Input: part model. Units: mm. Frame: model coordinates. Face numbers are marked on the shaded views. A direction names the side the tool comes from. Give positions to 0.01 mm unless a question says otherwise; leave off trailing zeros. Loops run counter-clockwise (first coordinate to the right, second up) from the corner with the lowest first, then second, coordinate; pieces in that order, holes last. Notation, with made-up numbers: (74.25, 3) - (115.25, 3) arc R26 cw to (115.25, 18) - close; hole circle Ø9 at (14, -13.5). An arc over 180 degrees is marked (long way). Answer as a JSON object with one key per item and string values.
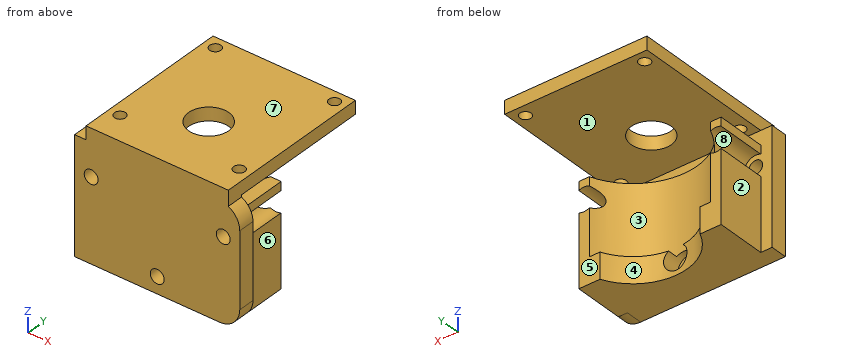
from build123d import *

# Parameters (mm, degrees)
SKETCH_1_W          = 30
SKETCH_1_H          = 30
EXTRUDE_1_DEPTH     = 5
SKETCH_2_W          = 30
SKETCH_2_H          = 5
EXTRUDE_2_DEPTH     = 10
SKETCH_3_R          = 2.1
CUT_EXTRUDE_1_DEPTH = 5
EXTRUDE_3_DEPTH     = 20
SKETCH_5_W          = 35
SKETCH_5_H          = 5
EXTRUDE_4_DEPTH     = 10
SKETCH_6_W          = 35
SKETCH_6_H          = 5
EXTRUDE_5_DEPTH     = 10
SKETCH_7_R          = 2.1
CUT_EXTRUDE_2_DEPTH = 10
FILLET_1_R          = 6.17
FILLET_2_R          = 6.17
SKETCH_8_W          = 43.093455854
SKETCH_8_H          = 31.755969384
CUT_EXTRUDE_3_DEPTH = 25
SKETCH_9_W          = 43.1
SKETCH_9_H          = 43.1
SKETCH_9_R          = 6.1
SKETCH_9_R_2        = 1.7
EXTRUDE_6_DEPTH     = 4
EXTRUDE_7_DEPTH     = 23
EXTRUDE_8_DEPTH     = 7.8
CUT_EXTRUDE_START   = -35
SKETCH_12_W         = 51.858978503
SKETCH_12_H         = 9.121001398
CUT_EXTRUDE_4_DEPTH = 35
SKETCH_14_W         = 43.1
SKETCH_14_H         = 5
EXTRUDE_9_DEPTH     = 8.2
SKETCH_15_R         = 2.1
CUT_EXTRUDE_5_DEPTH = 49.1
SKETCH_16_R         = 3.55
CUT_EXTRUDE_6_DEPTH = 44.1


with BuildPart() as part:
    # Sketch 1 → Extrude 1 (new body)
    with BuildSketch(Plane.XY):
        Rectangle(SKETCH_1_W, SKETCH_1_H)
    extrude(amount=EXTRUDE_1_DEPTH)

    # Sketch 2 → Extrude 2 (add)
    with BuildSketch(Plane(origin=(0, 0, 0), x_dir=(-1, 0, 0), z_dir=(0, 0, -1))):
        with Locations((0, -12.5)):
            Rectangle(SKETCH_2_W, SKETCH_2_H)
    extrude(amount=EXTRUDE_2_DEPTH)

    # Sketch 3 → Cut-Extrude 1 (cut)
    with BuildSketch(Plane(origin=(0, -10, 0), x_dir=(1, 0, 0), z_dir=(0, 1, 0))):
        with Locations((0, 5)):
            Circle(SKETCH_3_R)
    extrude(amount=-CUT_EXTRUDE_1_DEPTH, mode=Mode.SUBTRACT)

    # Sketch 4 → Extrude 3 (add)
    with BuildSketch(Plane.XY.offset(5)):
        Polygon((10.2, -15), (15, -15), (15, 15), (-15, 15), (-15, -15), (-10.2, -15), (-10.2, -18.997175384), (10.2, -18.997175384), align=None)
    extrude(amount=EXTRUDE_3_DEPTH)

    # Sketch 5 → Extrude 4 (add)
    with BuildSketch(Plane.ZY.offset(15)):
        with Locations((7.5, -12.5)):
            Rectangle(SKETCH_5_W, SKETCH_5_H)
    extrude(amount=EXTRUDE_4_DEPTH)

    # Sketch 6 → Extrude 5 (add)
    with BuildSketch(Plane(origin=(15, 0, 0), x_dir=(0, 0, -1), z_dir=(1, 0, 0))):
        with Locations((-7.5, -12.5)):
            Rectangle(SKETCH_6_W, SKETCH_6_H)
    extrude(amount=EXTRUDE_5_DEPTH)

    # Sketch 7 → Cut-Extrude 2 (cut)
    with BuildSketch(Plane(origin=(0, -10, 0), x_dir=(1, 0, 0), z_dir=(0, 1, 0))):
        with Locations((-20, -15)):
            Circle(SKETCH_7_R)
        with Locations((20, -15)):
            Circle(SKETCH_7_R)
    extrude(amount=-CUT_EXTRUDE_2_DEPTH, mode=Mode.SUBTRACT)

    # Fillet 1
    fillet_1_edges = [part.edges().sort_by_distance(p)[0] for p in [
        (25, -12.5, 25),
    ]]
    fillet(fillet_1_edges, radius=FILLET_1_R)

    # Fillet 2
    fillet_2_edges = [part.edges().sort_by_distance(p)[0] for p in [
        (25, -12.5, -10),
    ]]
    fillet(fillet_2_edges, radius=FILLET_2_R)

    # Sketch 8 → Cut-Extrude 3 (cut)
    with BuildSketch(Plane(origin=(0, 15, 0), x_dir=(1, 0, 0), z_dir=(0, 1, 0))):
        with Locations((-0.577881592, -10.851708682)):
            Rectangle(SKETCH_8_W, SKETCH_8_H)
    extrude(amount=-CUT_EXTRUDE_3_DEPTH, mode=Mode.SUBTRACT)

    # Sketch 12 → Cut-Extrude 4 (cut)
    with BuildSketch(Plane.XY.offset(25).offset(CUT_EXTRUDE_START)):
        with Locations((0.929489252, -19.560500699)):
            Rectangle(SKETCH_12_W, SKETCH_12_H)
    extrude(amount=CUT_EXTRUDE_4_DEPTH, mode=Mode.SUBTRACT)



with BuildPart() as body_2:
    # Sketch 9 → Extrude 6 (new body)
    with BuildSketch(Plane.XY.offset(29)):
        with Locations((0, 11.55)):
            Rectangle(SKETCH_9_W, SKETCH_9_H)
        with Locations((0, 4.5)):
            Circle(SKETCH_9_R, mode=Mode.SUBTRACT)
        with Locations((18.05, 29.6)):
            Circle(SKETCH_9_R_2, mode=Mode.SUBTRACT)
        with Locations((18.05, -6.5)):
            Circle(SKETCH_9_R_2, mode=Mode.SUBTRACT)
        with Locations((-18.05, -6.5)):
            Circle(SKETCH_9_R_2, mode=Mode.SUBTRACT)
        with Locations((-18.05, 29.6)):
            Circle(SKETCH_9_R_2, mode=Mode.SUBTRACT)
    extrude(amount=-EXTRUDE_6_DEPTH)


with BuildPart() as body_3:
    # Sketch 10 → Extrude 7 (new body)
    with BuildSketch(Plane(origin=(0, 0, 20.8), x_dir=(-1, 0, 0), z_dir=(0, 0, -1))):
        with BuildLine():
            Line((-21.55, 5), (-18.367022078, 5))
            ThreePointArc((-18.367022078, 5), (0, -7.95), (18.367022078, 5))
            Line((18.367022078, 5), (21.55, 5))
            Line((21.55, 5), (21.55, -10))
            Line((21.55, -10), (-21.55, -10))
            Line((-21.55, -10), (-21.55, 5))
        make_face()
    extrude(amount=EXTRUDE_7_DEPTH)

    # Sketch 11 → Extrude 8 (add)
    with BuildSketch(Plane(origin=(0, 0, -2.2), x_dir=(-1, 0, 0), z_dir=(0, 0, -1))):
        with BuildLine():
            Line((-21.55, 5), (-15.144223321, 5))
            ThreePointArc((-15.144223321, 5), (0, -4.95), (15.144223321, 5))
            Line((15.144223321, 5), (21.55, 5))
            Line((21.55, 5), (21.55, -10))
            Line((21.55, -10), (-21.55, -10))
            Line((-21.55, -10), (-21.55, 5))
        make_face()
    extrude(amount=EXTRUDE_8_DEPTH)


with BuildPart() as part_1:
    add(part.part)

    add(body_2.part)  # Extrude 9 merges body 2

    add(body_3.part)  # Extrude 9 merges body 3
    # Sketch 14 → Extrude 9 (add)
    with BuildSketch(Plane.XY.offset(29)):
        with Locations((0, -12.5)):
            Rectangle(SKETCH_14_W, SKETCH_14_H)
    extrude(amount=-EXTRUDE_9_DEPTH)

    # Sketch 15 → Cut-Extrude 5 (cut, through all)
    with BuildSketch(Plane.XZ.offset(15)):
        with Locations((-20, 15)):
            Circle(SKETCH_15_R)
        with Locations((0, -5)):
            Circle(SKETCH_15_R)
        with Locations((20, 15)):
            Circle(SKETCH_15_R)
    extrude(amount=-CUT_EXTRUDE_5_DEPTH, mode=Mode.SUBTRACT)

    # Sketch 16 → Cut-Extrude 6 (cut, through all)
    with BuildSketch(Plane(origin=(0, -10, 0), x_dir=(1, 0, 0), z_dir=(0, 1, 0))):
        with Locations((20, -15)):
            Circle(SKETCH_16_R)
        with Locations((0, 5)):
            Circle(SKETCH_16_R)
        with Locations((-20, -15)):
            Circle(SKETCH_16_R)
    extrude(amount=CUT_EXTRUDE_6_DEPTH, mode=Mode.SUBTRACT)


solid = part_1.part
Item 1: Access query for the marked faces 1, 2, 3, 4 and 5. Directions: +Z, -Z, +X, -X, +Y, -Y. A direction counts if a zero-diameter tool reaches every point of the face in a straight line with its end or side. Return the directions, or none.
Geometry check:
{"face 1": "+X, -X, +Y", "face 2": "+Z, -Z, -X, +Y", "face 3": "+Y", "face 4": "-Z, +Y", "face 5": "-Z, +X, -X, +Y"}
Item 2: Cut plane B-B (x = 0). Return loops of the section in (y, z), then the cut area to 3 significant figures.
Geometry check:
{"outline": "(-15, -10) - (-4.95, -10) - (-4.95, -8.55) - (-10, -8.55) - (-10, -7.1) - (-15, -7.1) - close; (-15, -2.9) - (-10, -2.9) - (-10, -1.45) - (-7.95, -1.45) - (-7.95, 20.8) - (-10, 20.8) - (-10, 25) - (-1.6, 25) - (-1.6, 29) - (-15, 29) - close; (10.6, 25) - (33.1, 25) - (33.1, 29) - (10.6, 29) - close", "area": "351 mm2"}
Item 3: Cut plane C-C (z = 15). Return loops of the section in (x, y).
Geometry check:
{"outline": "(-25, -15) - (-22.1, -15) - (-22.1, -10) - (-25, -10) - close; (-17.9, -15) - (17.9, -15) - (17.9, -10) - (16.45, -10) - (16.45, 1.08) arc R19.5 cw to (-16.45, 1.08) - (-16.45, -10) - (-17.9, -10) - close; (22.1, -15) - (25, -15) - (25, -10) - (22.1, -10) - close"}
Item 4: Material intervals for line 1 (Y direction, x = 18.05, z = 27.5); line 2 (Z direction, x = 20, y = -2); line 3 (X direction, y = -12, z = 15), sorted ascending. Write a range as [from, to].
Geometry check:
{"line 1": "y = [-15, -8.2], [-4.8, 27.9], [31.3, 33.1]", "line 2": "z = [-10, 11.45], [18.55, 20.8], [25, 29]", "line 3": "x = [-25, -22.1], [-17.9, 17.9], [22.1, 25]"}
Item 5: Contact query for flat-ended pins moving along their axis: P1, Ø3, axis at x = -23.5, y = -12, coming from the +Z side; P2, Ø12, axis at x = 2, y = 1, coming from the +Z side; P3, Ø0.8, axis at y = -5.5, z = 19.5, coming from the +X side; P4, Ø13, axis at x = -4.5, y = 21.5, coming from the -Z side. Output: stop coordinate, or through.
Geometry check:
{"P1": "stops at z = 25", "P2": "stops at z = 29", "P3": "stops at x = 21.55", "P4": "stops at z = 25"}
Item 6: Cut plane A-A (y = -9). Return loops of the section in (x, z).
Geometry check:
{"outline": "(-21.55, -10) - (21.55, -10) - (21.55, 11.81) arc R3.55 cw (long way) to (21.55, 18.19) - (21.55, 20.8) - (-21.55, 20.8) - (-21.55, 18.19) arc R3.55 cw (long way) to (-21.55, 11.81) - close; (-21.55, 25) - (21.55, 25) - (21.55, 29) - (-21.55, 29) - close; hole circle Ø7.1 at (0, -5)"}
Item 7: Mould query, pull axis X, two halves, no side actions, for the marked faces 6, 7 and 8. Classes: released by +X, released by -X, zero draft, split by the parting line, or undercut.
Geometry check:
{"face 6": "released by +X", "face 7": "zero draft", "face 8": "undercut"}
Item 8: Cut plane D-D (y = 2). Return loops of the section in (x, z).
Geometry check:
{"outline": "(-21.55, -10) - (-13.46, -10) - (-13.46, -2.2) - (-17, -2.2) - (-17, 13.1) arc R3.55 cw to (-21.55, 11.81) - close; (-21.55, 18.19) arc R3.55 cw to (-17, 16.9) - (-17, 20.8) - (-21.55, 20.8) - close; (-21.55, 25) - (-5.56, 25) - (-5.56, 29) - (-21.55, 29) - close; (5.56, 25) - (21.55, 25) - (21.55, 29) - (5.56, 29) - close; (13.46, -10) - (21.55, -10) - (21.55, 11.81) arc R3.55 cw to (17, 13.1) - (17, -2.2) - (13.46, -2.2) - close; (17, 16.9) arc R3.55 cw to (21.55, 18.19) - (21.55, 20.8) - (17, 20.8) - close"}
